Geometry check sheet. Reference: drawing and pictorial views, mm from the part's lowest x, y, z. Coordinates: 2 decimals unless noted, no trailing zeros. Write each loop counter-clockwise with the first axis right and the second up, starting at its lowest first coordinate (ties: lowest second). Pieces come first, ordered by that corner, then holes. Notation, with made-up numbers: (-6.5, 82) -> (33.5, 82) arc R19 ccw to (33.5, 105) -> close; hole circle Ø1 at (-19, -21.5). An arc over 180 degrees is marked (long way). Put each result on its own line as item: value.
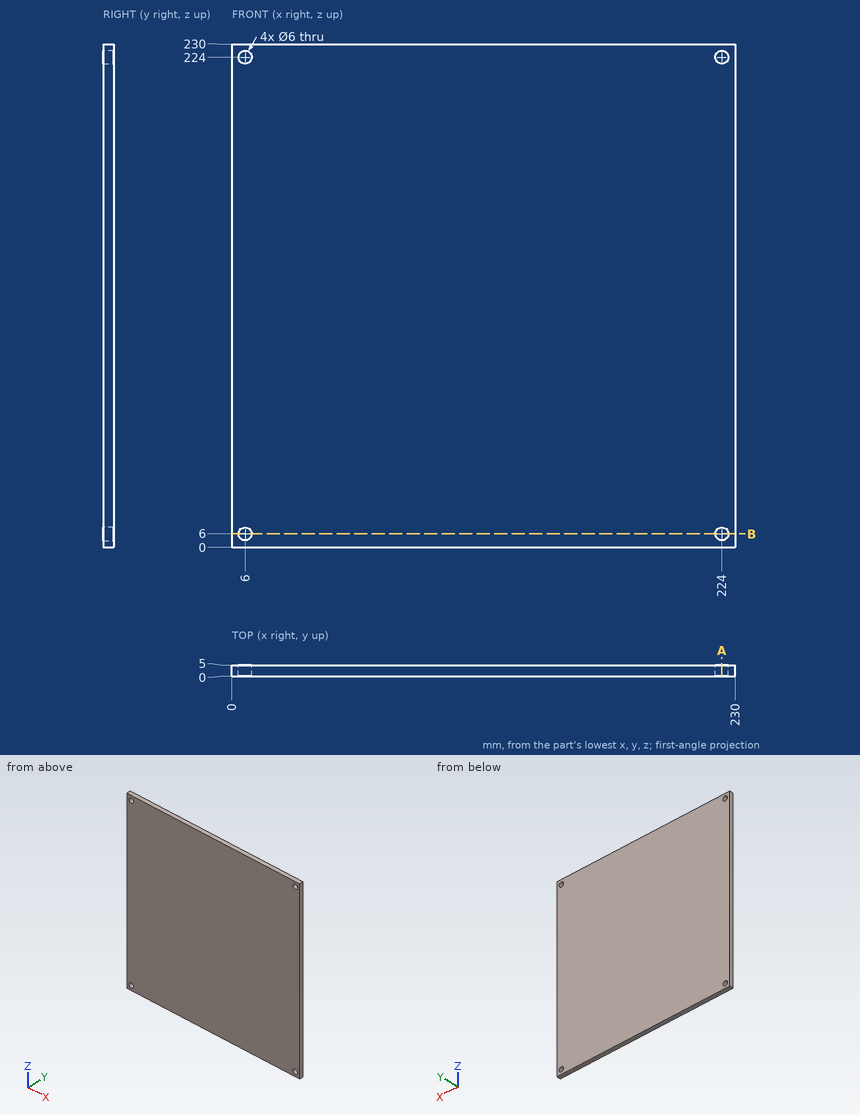
Q1. Cross-section at B-B (z = 6). Record the cut outline in (x, y).
Recorded:
outline: (0, 0) -> (3, 0) -> (3, 5) -> (0, 5) -> close; (9, 0) -> (221, 0) -> (221, 5) -> (9, 5) -> close; (227, 0) -> (230, 0) -> (230, 5) -> (227, 5) -> close
Q2. Cross-section at A-A (x = 224). Record the cut outline in (y, z).
Recorded:
outline: (0, 0) -> (5, 0) -> (5, 3) -> (0, 3) -> close; (0, 9) -> (5, 9) -> (5, 221) -> (0, 221) -> close; (0, 227) -> (5, 227) -> (5, 230) -> (0, 230) -> close
Q3. Depth check by flat-ended pin: P1, Ø5, axis at x = 201, z = 204.5, coming from the -Y side. Enter the tip coordinate at first touch or a pass-through.
Recorded:
P1: stops at y = 0
Q4. Material ranges on line 1 along X through (y, z) = (1.3, 6), recorded low to high.
Recorded:
line 1: x = 0 to 3, 9 to 221, 227 to 230
